Can you work these out from the drawing? Everything is in mm from the part's minimum corner. A direction names the side the tool comes from. Give positions to 0.01 mm unless a question says otherwise; leave off trailing zeros. Loops run counter-clockwise (first coordinate to the right, second up) from the corner with the lowest first, then second, coordinate; pieces in that order, holes last. Notation, with made-up numbers: M -23,84 L 20,84 A19 ccw 20,116 Z; hole C 64.25,-5 d7. An arc over 180 degrees is marked long. Use CSV: the item, a comma, the result in double quotes.
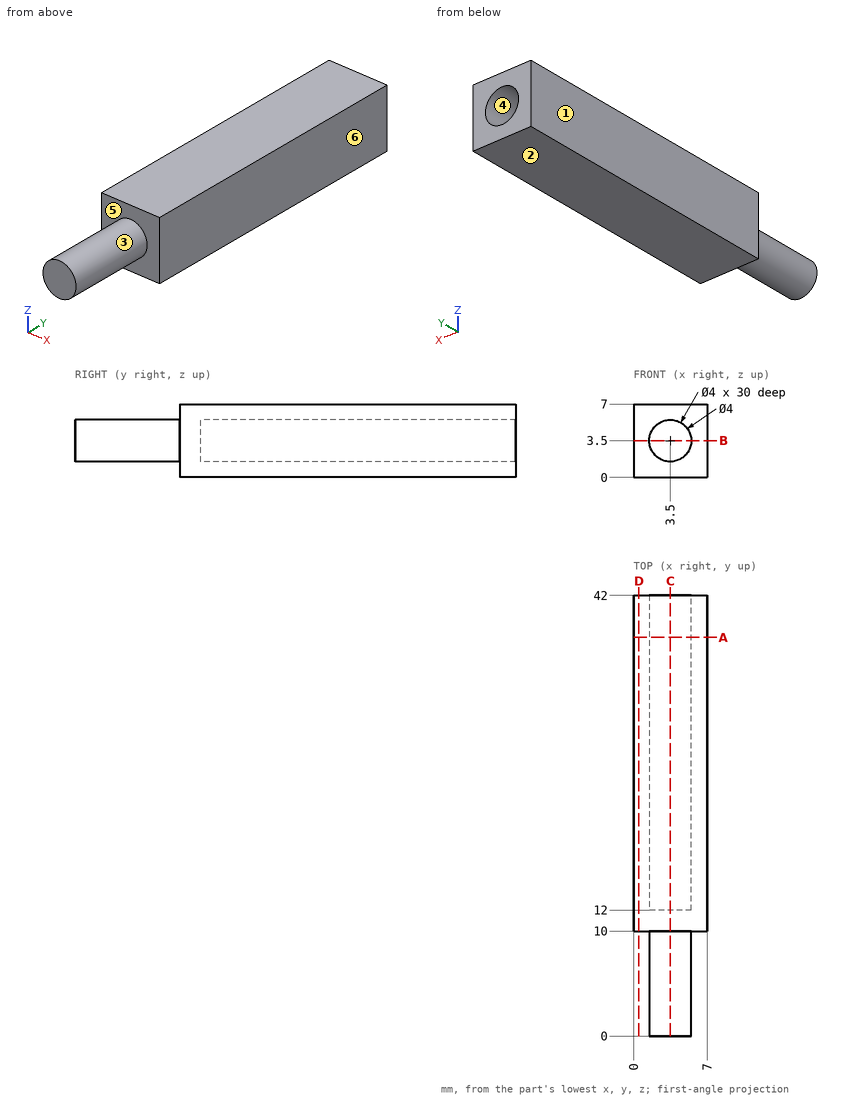
Q1. For the marked faces 5 and 6, which set-ups out of +Z, -Z, +X, -X, +Y, -Y let a thin tool reach every point of the face, with its end or its side?
Model answer:
face 5,"-Y"
face 6,"+Z, -Z, +X, +Y, -Y"
Q2. I want a section at D-D, the plane x = 0.5. Please give me the cut outline in (y, z), then the cut area to 3 significant figures.
Model answer:
outline,"M 10,0 L 42,0 L 42,7 L 10,7 Z"
area,"224 mm2"
Q3. Please list where these lines run through material, in increasing order: L1, parallel to X at y = 35.5, z = 3.5; L2, parallel to Y at x = 3.5, z = 6. Write a range as from..to.
Model answer:
L1,"0..1.5, 5.5..7"
L2,"10..42"
Q4. I want a section at A-A, the plane y = 38. Please give me the cut outline in (x, z), then the cut area to 3 significant figures.
Model answer:
outline,"M 0,0 L 7,0 L 7,7 L 0,7 Z; hole C 3.5,3.5 d4"
area,"36.4 mm2"
Q5. If we mould it in two halves opening along X, with no side actions, what happens to the marked faces 1, 2, 3 and 4? For each: released by +X, released by -X, zero draft, split by the parting line, or undercut.
Model answer:
face 1,"released by -X"
face 2,"zero draft"
face 3,"split by the parting line"
face 4,"undercut"
Q6. I want a section at B-B, the plane z = 3.5. Please give me the cut outline in (x, y), then the cut area to 3 significant figures.
Model answer:
outline,"M 0,10 L 1.5,10 L 1.5,0 L 5.5,0 L 5.5,10 L 7,10 L 7,42 L 5.5,42 L 5.5,12 L 1.5,12 L 1.5,42 L 0,42 Z"
area,"144 mm2"
Q7. I'm going to push flat-ended pins straight in: P1, Ø3, axis at x = 1.5, y = 29.5, coming from the -Z side; P2, Ø1.2, axis at x = 3.5, z = 4, coming from the +Y side; P3, Ø3, axis at x = 1.5, y = 4.5, coming from the +Z side. Where does each tip first touch, or does it pass through?
Model answer:
P1,"z = 0"
P2,"y = 12"
P3,"z = 5.44"
Q8. I want a section at C-C, the plane x = 3.5. Please give me the cut outline in (y, z), then the cut area to 3 significant figures.
Model answer:
outline,"M 0,1.5 L 10,1.5 L 10,0 L 42,0 L 42,1.5 L 12,1.5 L 12,5.5 L 42,5.5 L 42,7 L 10,7 L 10,5.5 L 0,5.5 Z"
area,"144 mm2"
